The model under review builds one solid part; all positions refer to its coordinate system, in mm. Coordinates: 2 decimals unless noted, no trailing zeros. Order: outer loops, then holes, each group sorted by start corner. A loop starts at its lowest first (then second) coordinate and runs counter-clockwise, first axis right, second up. Notation, with made-up numbers: (10, 69) - (32, 69) arc R6 cw to (32, 73) - close; hole circle Ø7 at (-0.75, 3.25). An arc over 180 degrees is marked (long way). Answer in a Markdown table with one row per item.
```python
from build123d import *

# Parameters (mm, degrees)
ESQUISSE2_R          = 0.5
BASE_EXTRUSION_DEPTH = 60


with BuildPart() as part:
    # Esquisse2 → Base-Extrusion (new body)
    with BuildSketch(Plane.XY):
        Circle(ESQUISSE2_R)
    extrude(amount=BASE_EXTRUSION_DEPTH)

    # Esquisse7 → Boss.-Révol.1 (revolve)
    with BuildSketch(Plane(origin=(0, 0, 0), x_dir=(1, 0, 0), z_dir=(0, 1, 0))):
        with BuildLine():
            Line((0, -60), (0, -60.5))
            ThreePointArc((0, -60.5), (-0.353553391, -60.353553391), (-0.5, -60))
            Line((-0.5, -60), (0, -60))
        make_face()
    revolve(axis=Axis((0, 0, 66.095405801), (0, 0, -1)))

    # Esquisse8 → Boss.-Révol.2 (revolve)
    with BuildSketch(Plane(origin=(0, 0, 0), x_dir=(1, 0, 0), z_dir=(0, 1, 0))):
        with BuildLine():
            Line((0, 0), (-0.5, 0))
            ThreePointArc((-0.5, 0), (-0.353553391, 0.353553391), (0, 0.5))
            Line((0, 0.5), (0, 0))
        make_face()
    revolve(axis=Axis((0, 0, -7.993801509), (0, 0, 1)))


solid = part.part
```
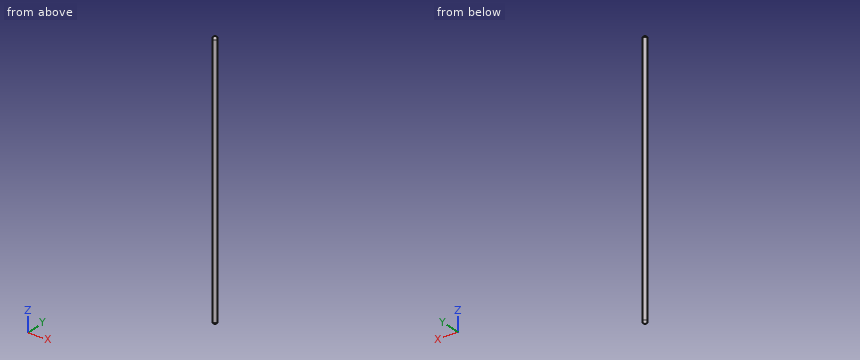
Item 1: We need section B-B, the plane x = -0.3. Write out the cut boundary in (y, z), then the cut area to 3 significant figures.
Check values:
| item | result |
|---|---|
| outline | (-0.4, 0) arc R0.4 ccw to (0.4, 0) - (0.4, 60) arc R0.4 ccw to (-0.4, 60) - close |
| area | 48.5 mm^2 |
Item 2: We need section A-A, the plane z = 6. Write out the cut boundary in (x, y), then the cut area to 3 significant figures.
Check values:
| item | result |
|---|---|
| outline | circle Ø1 at (0, 0) |
| area | 0.785 mm^2 |
Item 3: To check wall thickness, follow line 1 (Z direction, x = 0.1, y = -0.05); line 2 (X direction, y = 0.1, z = 31). State the ranges of each line that lie inside material, in increasing order. Write a range as from..to.
Check values:
| item | result |
|---|---|
| line 1 | -0.49..60.49 |
| line 2 | -0.49..0.49 |
Item 4: We need section C-C, the plane y = 0.2. Write out the cut boundary in (x, z).
Check values:
| item | result |
|---|---|
| outline | (-0.46, 0) arc R0.46 ccw to (0.46, 0) - (0.46, 60) arc R0.46 ccw to (-0.46, 60) - close |
